Here's how the part is built. I have some questions about the finished solid (model axes, mm). A direction names the side the tool comes from. Round coordinates to 2 decimals unless told otherwise and drop trailing zeros. Write each loop counter-clockwise with the first axis right and the second up, starting at its lowest first coordinate (ties: lowest second). Pieces come first, ordered by that corner, then holes. Notation, with made-up numbers: (47.25, 11.5) - (60.25, 11.5) arc R22 cw to (60.25, 23.5) - close; hole circle Ø9 at (-33.75, 4.5). An arc over 180 degrees is marked (long way). One line per item, written item: value. Start each with the question number.
Item 1: Thinking about a two-plate mould opening in X: for faces 1 (the face through (22.793, 96.86, -121.478)), 2 (the face through (24.627, -2.671, -0.14)), 3 (the face through (38.994, -13.812, -3.219)), which applies, released by +X, released by -X, zero draft, split by the parting line, or undercut?
Item 2: For P1, Ø4.5, axis at x = 72, y = 105.5, coming from the -Z side; P2, Ø6.5, axis at x = 71.51, z = -174.88, coming from the -Y side; P3, Ø4.5, axis at x = 72.5, y = 105.5, coming from the +Z side, each with a flat end and sliding along its axis, tell me the tip position at first contact or that it passes through.
Item 3: If I drill on line 1 (Z direction, x = 10.5, y = -6); line 2 (Y direction, x = 8.5, z = -92), over which ranges is the centre line in solid material (lowest first)?
Item 4: Imagine slicing it at B-B, the plane y = 10.5. Please give me the cut outline in (x, z), then the cut area to 3 significant figures.
Item 5: Imagine slicing it at A-A, the plane y = 90. Please give me the cut outline in (x, z), then the cut area to 3 significant figures.
Item 6: For faces 4 (the face through (30.79, -9.07, 0.03)), 5 (the face through (42.2, -15.66, -3.19)), 6 (the face through (35, 87, -111)), 7 (the face through (-10, 59, -8)), 8 (the face through (39.245, 96.86, -109.974)), which set-ups out of +Z, -Z, +X, -X, +Y, -Y let a thin tool reach every point of the face, with its end or its side?
Item 7: Imagine slicing it at C-C, the plane z = -105. Please give me the cut outline in (x, y), then the cut area to 3 significant figures.
```python
from build123d import *

# Parameters (mm, degrees)
SKETCH4_W           = 20
SKETCH4_H           = 20
SWEEP2_START        = -10
SWEEP2_OUTLINE_W    = 20
SWEEP2_OUTLINE_H    = 92
SWEEP2_DEPTH        = 20
SWEEP2_START_2      = -15
SWEEP2_2_OUTLINE_W  = 20
SWEEP2_2_OUTLINE_H  = 20
SWEEP2_2_DEPTH      = 5
SWEEP3_START        = 87
SWEEP3_DEPTH        = 20
CUT_EXTRUDE3_REACH  = 238.421
SKETCH5_R           = 2
SKETCH5_3_R         = 2
CUT_EXTRUDE4_DEPTH  = 5
CUT_EXTRUDE5_REACH  = 208.616
SKETCH6_R           = 2
SKETCH6_5_R         = 2
CUT_EXTRUDE6_DEPTH  = 5
CUT_EXTRUDE7_DEPTH  = 239.303090645
BOSS_EXTRUDE1_DEPTH = 20


# Read off the part's stored shape, not the designer's step: Sweep2, Sweep3
with BuildPart() as part:
    # Sweep1: sweep along a path in Sketch1
    with BuildLine(Plane.XY) as sweep1_path:
        Line((43.301270189, -25), (0, 0))
        Line((0, 0), (0, 15))
    # Sketch4 → Sweep1 (sweep)
    with BuildSketch(Plane(origin=(43.301270189, -25, 0), x_dir=(0, 0, -1), z_dir=(0.8660254037844382, -0.5000000000000011, 0))):
        Rectangle(SKETCH4_W, SKETCH4_H)
    sweep(path=sweep1_path.line, transition=Transition.RIGHT)

    # Sweep2 outline → Sweep2 (add)
    with BuildSketch(Plane.XY.offset(SWEEP2_START)):
        with Locations((0, 61)):
            Rectangle(SWEEP2_OUTLINE_W, SWEEP2_OUTLINE_H)
    extrude(amount=SWEEP2_DEPTH)

    # Sweep2 2 outline → Sweep2 2 (add)
    with BuildSketch(Plane.XY.offset(SWEEP2_START_2)):
        with Locations((0, 97)):
            Rectangle(SWEEP2_2_OUTLINE_W, SWEEP2_2_OUTLINE_H)
    extrude(amount=SWEEP2_2_DEPTH)

    # Sweep3 outline → Sweep3 (add)
    with BuildSketch(Plane(origin=(0, 0, 0), x_dir=(1, 0, 0), z_dir=(0, 1, 0)).offset(SWEEP3_START)):
        Polygon((54.679491924, 176.707658145), (-10, 64.679491924), (-10, 15), (10, 15), (10, 59.320508076), (69.320508076, 162.066641994), (96, 177.470053838), (86, 194.790561914), align=None)
    extrude(amount=SWEEP3_DEPTH)

    # Sketch5 → Cut-Extrude3 (cut, up to next)
    with BuildSketch(Plane(origin=(5, 8.660254038, 0), x_dir=(0.8660254037844382, -0.500000000000001, 0), z_dir=(0.5000000000000009, 0.866025403784438, 0)), mode=Mode.PRIVATE) as cut_extrude3_sk1:
        with Locations(Location((27.5, 0, 0), (0, 0, 180))):
            Circle(SKETCH5_R)
    cut_extrude3_tool1 = extrude(cut_extrude3_sk1.sketch, amount=-CUT_EXTRUDE3_REACH, mode=Mode.PRIVATE) & part.part
    # Sketch5 → Cut-Extrude3 (cut, up to next)
    with BuildSketch(Plane(origin=(5, 8.660254038, 0), x_dir=(0.8660254037844382, -0.500000000000001, 0), z_dir=(0.5000000000000009, 0.866025403784438, 0)), mode=Mode.PRIVATE) as cut_extrude3_sk2:
        with Locations(Location((42.5, 0, 0), (0, 0, 180))):
            Circle(SKETCH5_R)
    cut_extrude3_tool2 = extrude(cut_extrude3_sk2.sketch, amount=-CUT_EXTRUDE3_REACH, mode=Mode.PRIVATE) & part.part
    add(cut_extrude3_tool1.solids().sort_by_distance((28.815699, -5.089746, 0))[0], mode=Mode.SUBTRACT)
    add(cut_extrude3_tool2.solids().sort_by_distance((41.80608, -12.589746, 0))[0], mode=Mode.SUBTRACT)

    # Sketch5<3> → Cut-Extrude4 (cut)
    # profile 1 of 2: a face of its own
    with BuildSketch(Plane(origin=(5, 8.660254038, 0), x_dir=(0.8660254037844382, -0.500000000000001, 0), z_dir=(0.5000000000000009, 0.866025403784438, 0))):
        Polygon((31.2, -2.136195996), (31.2, 2.136195996), (27.5, 4.272391992), (23.8, 2.136195996), (23.8, -2.136195996), (27.5, -4.272391992), align=None)
        with Locations(Location((27.5, 0, 0), (0, 0, 180))):
            Circle(SKETCH5_3_R, mode=Mode.SUBTRACT)
    # profile 2 of 2: a face of its own
    with BuildSketch(Plane(origin=(5, 8.660254038, 0), x_dir=(0.8660254037844382, -0.500000000000001, 0), z_dir=(0.5000000000000009, 0.866025403784438, 0))):
        Polygon((46.2, -2.136195996), (46.2, 2.136195996), (42.5, 4.272391992), (38.8, 2.136195996), (38.8, -2.136195996), (42.5, -4.272391992), align=None)
        with Locations(Location((42.5, 0, 0), (0, 0, 180))):
            Circle(SKETCH5_3_R, mode=Mode.SUBTRACT)
    extrude(amount=-CUT_EXTRUDE4_DEPTH, mode=Mode.SUBTRACT)

    # Sketch6 → Cut-Extrude5 (cut, up to next)
    with BuildSketch(Plane(origin=(0, 107, -107), x_dir=(1, 0, 0), z_dir=(0, -1, 0)), mode=Mode.PRIVATE) as cut_extrude5_sk1:
        with Locations(Location((71.514428415, -67.880307876, 0), (0, 0, 90))):
            Circle(SKETCH6_R)
    cut_extrude5_tool1 = extrude(cut_extrude5_sk1.sketch, amount=CUT_EXTRUDE5_REACH, mode=Mode.PRIVATE) & part.part
    # Sketch6 → Cut-Extrude5 (cut, up to next)
    with BuildSketch(Plane(origin=(0, 107, -107), x_dir=(1, 0, 0), z_dir=(0, -1, 0)), mode=Mode.PRIVATE) as cut_extrude5_sk2:
        with Locations(Location((84.504809472, -75.380307876, 0), (0, 0, 90))):
            Circle(SKETCH6_R)
    cut_extrude5_tool2 = extrude(cut_extrude5_sk2.sketch, amount=CUT_EXTRUDE5_REACH, mode=Mode.PRIVATE) & part.part
    add(cut_extrude5_tool1.solids().sort_by_distance((71.514428, 107, -174.880308))[0], mode=Mode.SUBTRACT)
    add(cut_extrude5_tool2.solids().sort_by_distance((84.504809, 107, -182.380308))[0], mode=Mode.SUBTRACT)

    # Sketch6<5> → Cut-Extrude6 (cut)
    # profile 1 of 2: a face of its own
    with BuildSketch(Plane(origin=(0, 107, -107), x_dir=(1, 0, 0), z_dir=(0, -1, 0))):
        Polygon((75.786820407, -67.880307876), (73.650624411, -64.180307876), (69.378232419, -64.180307876), (67.242036423, -67.880307876), (69.378232419, -71.580307876), (73.650624411, -71.580307876), align=None)
        with Locations(Location((71.514428415, -67.880307876, 0), (0, 0, 90))):
            Circle(SKETCH6_5_R, mode=Mode.SUBTRACT)
    # profile 2 of 2: a face of its own
    with BuildSketch(Plane(origin=(0, 107, -107), x_dir=(1, 0, 0), z_dir=(0, -1, 0))):
        Polygon((88.777201464, -75.380307876), (86.641005468, -71.680307876), (82.368613476, -71.680307876), (80.23241748, -75.380307876), (82.368613476, -79.080307876), (86.641005468, -79.080307876), align=None)
        with Locations(Location((84.504809472, -75.380307876, 0), (0, 0, 90))):
            Circle(SKETCH6_5_R, mode=Mode.SUBTRACT)
    extrude(amount=CUT_EXTRUDE6_DEPTH, mode=Mode.SUBTRACT)

    # Sketch7 → Cut-Extrude7 (cut, through all)
    with BuildSketch(Plane(origin=(10, 0, 0), x_dir=(0, 0, -1), z_dir=(1, 0, 0))):
        Polygon((4.356747298, 92.643252702), (-10, 107), (-10, 78.286505404), align=None)
        Polygon((18.713494596, 107), (-10, 107), (4.356747298, 92.643252702), align=None)
    extrude(amount=-CUT_EXTRUDE7_DEPTH, mode=Mode.SUBTRACT)

    # Sketch7<3> → Boss-Extrude1 (add, through all)
    with BuildSketch(Plane(origin=(10, 0, 0), x_dir=(0, 0, -1), z_dir=(1, 0, 0))):
        Polygon((26.997765843, 87), (10, 87), (10, 70.002234157), align=None)
    extrude(amount=-BOSS_EXTRUDE1_DEPTH)


solid = part.part
```
Values follow:
1. face 1: released by -X
1. face 2: released by +X
1. face 3: undercut
2. P1: stops at z = -188.01
2. P2: stops at y = 87
2. P3: stops at z = -162.6
3. line 1: z = -10 to 10
3. line 2: y = 87 to 107
4. outline: (-10, -10) - (10, -10) - (10, 10) - (-10, 10) - close
4. area: 400 mm^2
5. outline: (-10, -64.68) - (54.68, -176.71) - (86, -194.79) - (96, -177.47) - (69.32, -162.07) - (10, -59.32) - (10, -1.71) - (-10, -1.71) - close; hole circle Ø4 at (71.51, -174.88); hole circle Ø4 at (84.5, -182.38)
5. area: 4,330 mm^2
6. face 4: +Y
6. face 5: none
6. face 6: -Z, +X, -X, -Y
6. face 7: +Z, -Z, -X, +Y, -Y
6. face 8: +Z, +X, +Y, -Y
7. outline: (13.28, 87) - (36.37, 87) - (36.37, 107) - (13.28, 107) - close
7. area: 462 mm^2
